Here's the drawing with two shaded views (mm, measured from the low corner). I have some questions. A direction names the side the tool comes from. Give positions to 0.01 mm unless a question says otherwise; leave off trailing zeros. Loops run counter-clockwise (first coordinate to the right, second up) from the corner with the lowest first, then second, coordinate; pieces in that order, holes last. Notation, with made-up numbers: M 24.5,55 L 83.5,55 A25 cw 83.5,91 Z; hole C 52,62 d2. An arc over 180 degrees is marked long. Use CSV: the item, a comma, the result in double quotes.
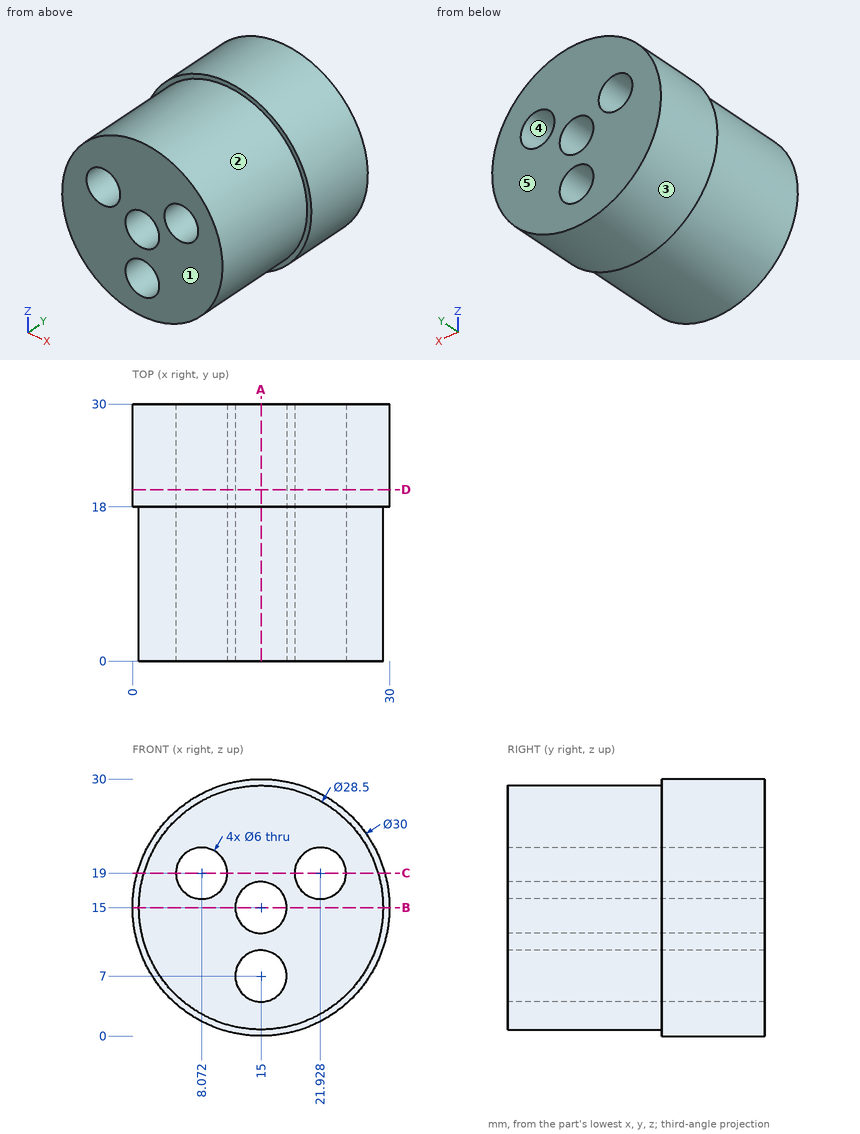
1. If we mould it in two halves opening along X, with no side actions, what happens to the marked faces 3, 4 and 5? For each: +X half, -X half, draft (parallel to the pull), parting line (faces both ways), or undercut.
Outcome:
face 3,"parting line"
face 4,"undercut"
face 5,"draft"
2. I want a section at B-B, the plane z = 15. List the corners of the cut face in (x, y) for me.
Outcome:
outline,"M 0,18 L 0.75,18 L 0.75,0 L 12,0 L 12,30 L 0,30 Z; M 18,0 L 29.25,0 L 29.25,18 L 30,18 L 30,30 L 18,30 Z"
3. Which directions (+Z, -Z, +X, -X, +Y, -Y) give clear straight access to the entire face, cutting with the end or side of a thin tool? Please do the marked faces 1 and 2.
Outcome:
face 1,"+Z, -Z, +X, -X, -Y"
face 2,"-Y"
4. I'm going to push flat-ended pins straight in: pin 1 Ø3 at (y, z) = (25, 6.5) entering from +X; pin 2 Ø5 at (y, z) = (10, 11) entering from +X; pin 3 Ø5 at (y, z) = (27, 22) entering from +X. Where does each tip first touch, or does it pass through?
Outcome:
pin 1,"x = 28.27"
pin 2,"x = 29.17"
pin 3,"x = 29.31"
5. I want a section at C-C, the plane z = 19. List the corners of the cut face in (x, y) for me.
Outcome:
outline,"M 0.54,18 L 1.32,18 L 1.32,0 L 5.07,0 L 5.07,30 L 0.54,30 Z; M 11.07,0 L 18.93,0 L 18.93,30 L 11.07,30 Z; M 24.93,0 L 28.68,0 L 28.68,18 L 29.46,18 L 29.46,30 L 24.93,30 Z"
6. I want a section at A-A, the plane x = 15. List the corners of the cut face in (y, z) for me.
Outcome:
outline,"M 0,0.75 L 18,0.75 L 18,0 L 30,0 L 30,4 L 0,4 Z; M 0,10 L 30,10 L 30,12 L 0,12 Z; M 0,18 L 30,18 L 30,30 L 18,30 L 18,29.25 L 0,29.25 Z"
7. I want a section at D-D, the plane y = 20. List the corners of the cut face in (x, z) for me.
Outcome:
outline,"C 15,15 d30; hole C 8.07,19 d6; hole C 15,7 d6; hole C 15,15 d6; hole C 21.93,19 d6"
8. Please list where these lines run through material, in increasing order: line 1 (Z direction, x = 17.5, y = 15.75); line 2 (Z direction, x = 13, y = 19.75) (1 decimal); line 3 (X direction, y = 20.25, z = 19.5).
Outcome:
line 1,"0.97 to 5.34, 8.66 to 13.34, 16.66 to 29.03"
line 2,"0.1 to 4.8, 9.2 to 12.8, 17.2 to 29.9"
line 3,"0.69 to 5.11, 11.03 to 18.97, 24.89 to 29.31"
